```python
from build123d import *

# Parameters (mm, degrees)
EXTRUDE_1_DEPTH     = 8
EXTRUDE_2_DEPTH     = 8
CUT_EXTRUDE_1_REACH = 83.388
SKETCH_3_R          = 4
CUT_EXTRUDE_2_REACH = 100.224
SKETCH_4_R          = 4


with BuildPart() as part:
    # 草图1 → 凸台-拉伸1 (new body)
    with BuildSketch(Plane.XY):
        with BuildLine():
            Line((-20, 20), (20, 20))
            Line((20, 20), (20, -20))
            ThreePointArc((20, -20), (0, -40), (-20, -20))
            Line((-20, -20), (-20, 20))
        make_face()
    extrude(amount=EXTRUDE_1_DEPTH)

    # 草图2 → 凸台-拉伸2 (add)
    with BuildSketch(Plane(origin=(0, 20, 0), x_dir=(1, 0, 0), z_dir=(0, 1, 0))):
        with BuildLine():
            Line((-20, 0), (20, 0))
            Line((20, 0), (20, -48))
            ThreePointArc((20, -48), (0, -68), (-20, -48))
            Line((-20, -48), (-20, 0))
        make_face()
    extrude(amount=EXTRUDE_2_DEPTH)

    # 草图3 → 切除-拉伸1 (cut, up to next)
    with BuildSketch(Plane(origin=(0, 0, 0), x_dir=(-1, 0, 0), z_dir=(0, 0, -1)), mode=Mode.PRIVATE) as cut_extrude_1_sk1:
        with Locations((-10, -2)):
            Circle(SKETCH_3_R)
    cut_extrude_1_tool1 = extrude(cut_extrude_1_sk1.sketch, amount=-CUT_EXTRUDE_1_REACH, mode=Mode.PRIVATE) & part.part
    # 草图3 → 切除-拉伸1 (cut, up to next)
    with BuildSketch(Plane(origin=(0, 0, 0), x_dir=(-1, 0, 0), z_dir=(0, 0, -1)), mode=Mode.PRIVATE) as cut_extrude_1_sk2:
        with Locations((10, -2)):
            Circle(SKETCH_3_R)
    cut_extrude_1_tool2 = extrude(cut_extrude_1_sk2.sketch, amount=-CUT_EXTRUDE_1_REACH, mode=Mode.PRIVATE) & part.part
    add(cut_extrude_1_tool1.solids().sort_by_distance((10, -2, 0))[0], mode=Mode.SUBTRACT)
    add(cut_extrude_1_tool2.solids().sort_by_distance((-10, -2, 0))[0], mode=Mode.SUBTRACT)

    # 草图4 → 切除-拉伸2 (cut, up to next)
    with BuildSketch(Plane(origin=(0, 28, 0), x_dir=(1, 0, 0), z_dir=(0, 1, 0)), mode=Mode.PRIVATE) as cut_extrude_2_sk1:
        with Locations(Location((-10, -30, 0), (0, 0, 270))):
            Circle(SKETCH_4_R)
    cut_extrude_2_tool1 = extrude(cut_extrude_2_sk1.sketch, amount=-CUT_EXTRUDE_2_REACH, mode=Mode.PRIVATE) & part.part
    # 草图4 → 切除-拉伸2 (cut, up to next)
    with BuildSketch(Plane(origin=(0, 28, 0), x_dir=(1, 0, 0), z_dir=(0, 1, 0)), mode=Mode.PRIVATE) as cut_extrude_2_sk2:
        with Locations(Location((10, -30, 0), (0, 0, 270))):
            Circle(SKETCH_4_R)
    cut_extrude_2_tool2 = extrude(cut_extrude_2_sk2.sketch, amount=-CUT_EXTRUDE_2_REACH, mode=Mode.PRIVATE) & part.part
    add(cut_extrude_2_tool1.solids().sort_by_distance((-10, 28, 30))[0], mode=Mode.SUBTRACT)
    add(cut_extrude_2_tool2.solids().sort_by_distance((10, 28, 30))[0], mode=Mode.SUBTRACT)


solid = part.part
```
Design review of the part built by this model. Coordinates are the model's own, in mm. A direction names the side the tool comes from. Round coordinates to 2 decimals unless told otherwise and drop trailing zeros. Write each loop counter-clockwise with the first axis right and the second up, starting at its lowest first coordinate (ties: lowest second). Pieces come first, ordered by that corner, then holes.
Item 1: We need section C-C on x = -10. Write out the cut boundary in (y, z), and give its area (3 significant figures).
Item 2: The part is to be moulded in two halves that separate along X. For faces 3 (the flat face through (20, 13, 6)), 4 (the cylindrical face through (14, -2, 4)), 5 (the cylindrical face through (-12.4, 24.1, 26.8)), 6 (the flat face through (-20, 13, 6)), say which applies: +X half, -X half, draft (parallel to the pull), parting line (faces both ways), or undercut.
Item 3: Clearance check with flat-ended pins moving along their axes: pin 1 Ø6 at (x, y) = (11.5, 14) entering from +Z; pin 2 Ø5 at (x, z) = (3.5, 10) entering from -Y; pin 3 Ø5 at (x, y) = (-6, -29.5) entering from -Z. State where each tip first meets the part, or that it passes through.
Item 4: For probe 1 along X at (y, z) = (24, 30); probe 2 along Z at (x, y) = (-13, -28); probe 3 along Y at (x, z) = (-14.5, 53.5), list the stretches that pass through material, from the lowest coordinate up.
Item 5: For faces 1 (the flat face through (0, -6, 0)), 2 (the flat face through (0, -10, 8)), list the 3-axis set-ups (+Z, -Z, +X, -X, +Y, -Y) from which the entire face can be reached by the end or side of a thin tool; tool diameter is ignored.
Item 6: We need section B-B on z = 30. Write out the cut boundary in (x, y).
Item 7: We need section D-D on z = 5. Write out the cut boundary in (x, y), and give its area (3 significant figures).
Item 8: We need section A-A on y = -2. Write out the cut boundary in (x, z), and give its area (3 significant figures).
Returned:
1. outline: (-37.32, 0) - (-6, 0) - (-6, 8) - (-37.32, 8) - close; (2, 0) - (28, 0) - (28, 26) - (20, 26) - (20, 8) - (2, 8) - close; (20, 34) - (28, 34) - (28, 65.32) - (20, 65.32) - close
1. area: 853 mm2
2. face 3: +X half
2. face 4: undercut
2. face 5: undercut
2. face 6: -X half
3. pin 1: stops at z = 8
3. pin 2: stops at y = -39.9
3. pin 3: stops at z = 0
4. probe 1: x = -20 to -14, -6 to 6, 14 to 20
4. probe 2: z = 0 to 8
4. probe 3: y = 20 to 28
5. face 1: -Z, +X, -X, +Y, -Y
5. face 2: +Z, +X, -X, -Y
6. outline: (-20, 20) - (-14, 20) - (-14, 28) - (-20, 28) - close; (-6, 20) - (6, 20) - (6, 28) - (-6, 28) - close; (14, 20) - (20, 20) - (20, 28) - (14, 28) - close
7. outline: (-20, -20) arc R20 ccw to (20, -20) - (20, 28) - (-20, 28) - close; hole circle Ø8 at (-10, -2); hole circle Ø8 at (10, -2)
7. area: 2,450 mm2
8. outline: (-20, 0) - (-14, 0) - (-14, 8) - (-20, 8) - close; (-6, 0) - (6, 0) - (6, 8) - (-6, 8) - close; (14, 0) - (20, 0) - (20, 8) - (14, 8) - close
8. area: 192 mm2
